Source: CAD feature listing. Evaluate the final solid. Frame: model axes, mm. Face numbers are marked on the shaded views. A direction names the side the tool comes from. Round coordinates to 2 decimals unless told otherwise and drop trailing zeros. Order: outer loops, then holes, each group sorted by start corner. A loop starts at its lowest first (then second) coordinate and runs counter-clockwise, first axis right, second up. Notation, with made-up numbers: M 20.5,33 L 49.5,33 A4 cw 49.5,40 Z; hole C 46,-30.5 d10. An arc over 180 degrees is marked long. Use one line per item in the form item = value. Start each with the question number.
Q1. Contact query for flat-ended pins moving along their axis: pin 1 (2.5 mm diameter, centred on x = 226, z = -75, fed in from +Y); pin 2 (1 mm diameter, centred on x = 87, z = -62, fed in from +Y); pin 3 (22 mm diameter, centred on x = 203.5, y = 2.5, fed in from +Z). Output: stop coordinate, or through.
Q2. Pull-direction query (X, two-part tool) for the marked faces 4, 5, 6 and 7; classes: pulls with the +X half, pulls with the -X half, needs draft (parallel to the pull), parting line crosses it, or undercut.
Q3. Reachability of the marked faces 1, 2 and 3 from +Z, -Z, +X, -X, +Y, -Y: full face, straight path, thin tool, end or side. Return the list, or none.
Q4. Section D-D (x = 185). Return the cut outline in (y, z), plus the area to 3 significant figures.
Q5. Section B-B (y = 4.5). Return the cut outline in (x, z).
Q6. Section A-A (z = 45.5). Return the cut outline in (x, y).
Q7. Material intervals for probe 1 along X at (y, z) = (9, -29); probe 2 along Z at (x, y) = (111, 26.5); probe 3 along X at (y, z) = (13.5, 72.5), sorted ascending.
Q8. Section C-C (y = 17.5). Return the cut outline in (x, z).
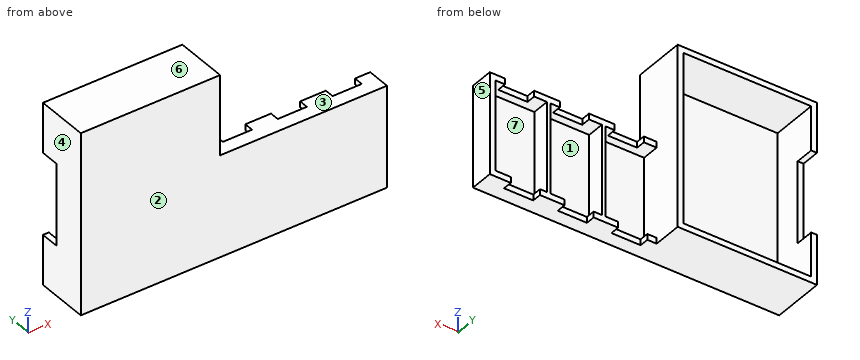
from build123d import *

# Parameters (mm, degrees)
BOSS_EXTRUDE1_DEPTH = 40
BOSS_EXTRUDE2_DEPTH = 5
SKETCH4_W           = 5
SKETCH4_H           = 77
SKETCH4_W_2         = 3
BOSS_EXTRUDE3_DEPTH = 40
SKETCH5_W           = 143
SKETCH5_H           = 87
CUT_EXTRUDE1_DEPTH  = 25
SKETCH6_W           = 25
SKETCH6_H           = 5
CUT_EXTRUDE2_DEPTH  = 8
SKETCH7_W           = 5
SKETCH7_H           = 70
CUT_EXTRUDE3_DEPTH  = 16


with BuildPart() as part:
    # Sketch1 → Boss-Extrude1 (new body)
    with BuildSketch(Plane(origin=(0, 0, 0), x_dir=(1, 0, 0), z_dir=(0, 1, 0))):
        Polygon((0, 77.75), (0, -77.75), (119.4, -77.75), (119.4, -9.25), (262.4, -9.25), (262.4, 77.75), align=None)
        Polygon((5, 72.75), (257.4, 72.75), (257.4, -4.25), (114.4, -4.25), (114.4, -72.75), (5, -72.75), align=None, mode=Mode.SUBTRACT)
    extrude(amount=BOSS_EXTRUDE1_DEPTH)

    # Sketch3 → Boss-Extrude2 (add)
    with BuildSketch(Plane.XZ):
        Polygon((119.4, 77.75), (119.4, 9.25), (262.4, 9.25), (262.4, -77.75), (0, -77.75), (0, 77.75), align=None)
    extrude(amount=BOSS_EXTRUDE2_DEPTH)

    # Sketch4 → Boss-Extrude3 (add)
    with BuildSketch(Plane(origin=(0, 0, 0), x_dir=(1, 0, 0), z_dir=(0, 1, 0))):
        with Locations((116.9, 34.25)):
            Rectangle(SKETCH4_W, SKETCH4_H)
        with Locations((164.9, 34.25)):
            Rectangle(SKETCH4_W_2, SKETCH4_H)
        with Locations((211.9, 34.25)):
            Rectangle(SKETCH4_W_2, SKETCH4_H)
    extrude(amount=BOSS_EXTRUDE3_DEPTH)

    # Sketch5 → Cut-Extrude1 (cut)
    with BuildSketch(Plane(origin=(0, 40, 0), x_dir=(1, 0, 0), z_dir=(0, 1, 0))):
        with Locations((190.9, 34.25)):
            Rectangle(SKETCH5_W, SKETCH5_H)
    extrude(amount=-CUT_EXTRUDE1_DEPTH, mode=Mode.SUBTRACT)

    # Sketch6 → Cut-Extrude2 (cut)
    with BuildSketch(Plane(origin=(0, 15, 0), x_dir=(1, 0, 0), z_dir=(0, 1, 0))):
        with Locations((142.9, -6.75)):
            Rectangle(SKETCH6_W, SKETCH6_H)
        with Locations((189.9, -6.75)):
            Rectangle(SKETCH6_W, SKETCH6_H)
        with Locations((236.9, -6.75)):
            Rectangle(SKETCH6_W, SKETCH6_H)
        with Locations((139.9, 75.25)):
            Rectangle(SKETCH6_W, SKETCH6_H)
        with Locations((185.9, 75.25)):
            Rectangle(SKETCH6_W, SKETCH6_H)
        with Locations((231.9, 75.25)):
            Rectangle(SKETCH6_W, SKETCH6_H)
    extrude(amount=-CUT_EXTRUDE2_DEPTH, mode=Mode.SUBTRACT)

    # Sketch7 → Cut-Extrude3 (cut)
    with BuildSketch(Plane(origin=(0, 40, 0), x_dir=(1, 0, 0), z_dir=(0, 1, 0))):
        with Locations((2.5, 0)):
            Rectangle(SKETCH7_W, SKETCH7_H)
    extrude(amount=-CUT_EXTRUDE3_DEPTH, mode=Mode.SUBTRACT)


solid = part.part
Results list:
q1.pin_1 = 7
q1.pin_2 = 0
q1.pin_3 = 9.25
q2.face_4 = pulls with the -X half
q2.face_5 = pulls with the +X half
q2.face_6 = needs draft
q2.face_7 = undercut
q3.face_1 = +Y
q3.face_2 = +Z, -Z, +X, -X, -Y
q3.face_3 = +Z, +X, +Y, -Y
q4.outline = M -5,-77.75 L 7,-77.75 L 7,-72.75 L 0,-72.75 L 0,4.25 L 7,4.25 L 7,9.25 L -5,9.25 Z
q4.area = 505 mm2
q5.outline = M 0,-77.75 L 262.4,-77.75 L 262.4,9.25 L 119.4,9.25 L 119.4,77.75 L 0,77.75 Z; hole M 5,-72.75 L 114.4,-72.75 L 114.4,72.75 L 5,72.75 Z; hole M 119.4,-72.75 L 163.4,-72.75 L 163.4,4.25 L 119.4,4.25 Z; hole M 166.4,-72.75 L 210.4,-72.75 L 210.4,4.25 L 166.4,4.25 Z; hole M 213.4,-72.75 L 257.4,-72.75 L 257.4,4.25 L 213.4,4.25 Z
q6.outline = M 0,-5 L 119.4,-5 L 119.4,40 L 114.4,40 L 114.4,0 L 5,0 L 5,40 L 0,40 Z
q7.probe_1 = 0 to 5, 114.4 to 119.4, 163.4 to 166.4, 210.4 to 213.4, 257.4 to 262.4
q7.probe_2 = -77.75 to -72.75, 72.75 to 77.75
q7.probe_3 = 0 to 5, 114.4 to 119.4
q8.outline = M 0,-77.75 L 119.4,-77.75 L 119.4,77.75 L 0,77.75 Z; hole M 5,-72.75 L 114.4,-72.75 L 114.4,72.75 L 5,72.75 Z
